Verification items for this drawing (mm, ordinates from the low corner). A direction names the side the tool comes from. Round coordinates to 2 decimals unless told otherwise and drop trailing zeros. Order: outer loops, then holes, each group sorted by start corner. A loop starts at its lowest first (then second) coordinate and runs counter-clockwise, first axis right, second up. Notation, with made-up numbers: (26, -37.5) - (42, -37.5) arc R12 ccw to (42, -32.5) - close; hole circle Ø6 at (48, 21). An arc over 180 degrees is marked (long way). Return JSON: item names as keys, results as strings. Group by question number.
Q1. Sectioned sample at A-A, the plane z = 9.5. Record the cut outline in (x, y).
Q2. Material ranges on line 1 along Y through (x, z) = (3, 14); line 2 along Z through (x, y) = (3.7, 0.5); line 3 along Z through (x, y) = (3.8, 2.35), recorded low to high.
Q3. Tool access check on the marked faces 1 and 2. Record the directions out of +Z, -Z, +X, -X, +Y, -Y that give a thin tool (end or side, any length) a straight path to the whole face; none if there is none.
Q4. Sectioned sample at D-D, the plane y = 4.35. Record the cut outline in (x, z), then the cut area to 3 significant figures.
Q5. Sectioned sample at C-C, the plane y = 2.05. Record the cut outline in (x, z).
Q6. Sectioned sample at B-B, the plane x = 3. Record the cut outline in (y, z).
Q7. Gauge pin test, flat ends, axial feed: pin 1 Ø0.8 at (x, y) = (3, 2.5) entering from -Z; pin 2 Ø2 at (x, y) = (1, 4) entering from +Z. Record the tip position at first contact, or that the pin passes through.
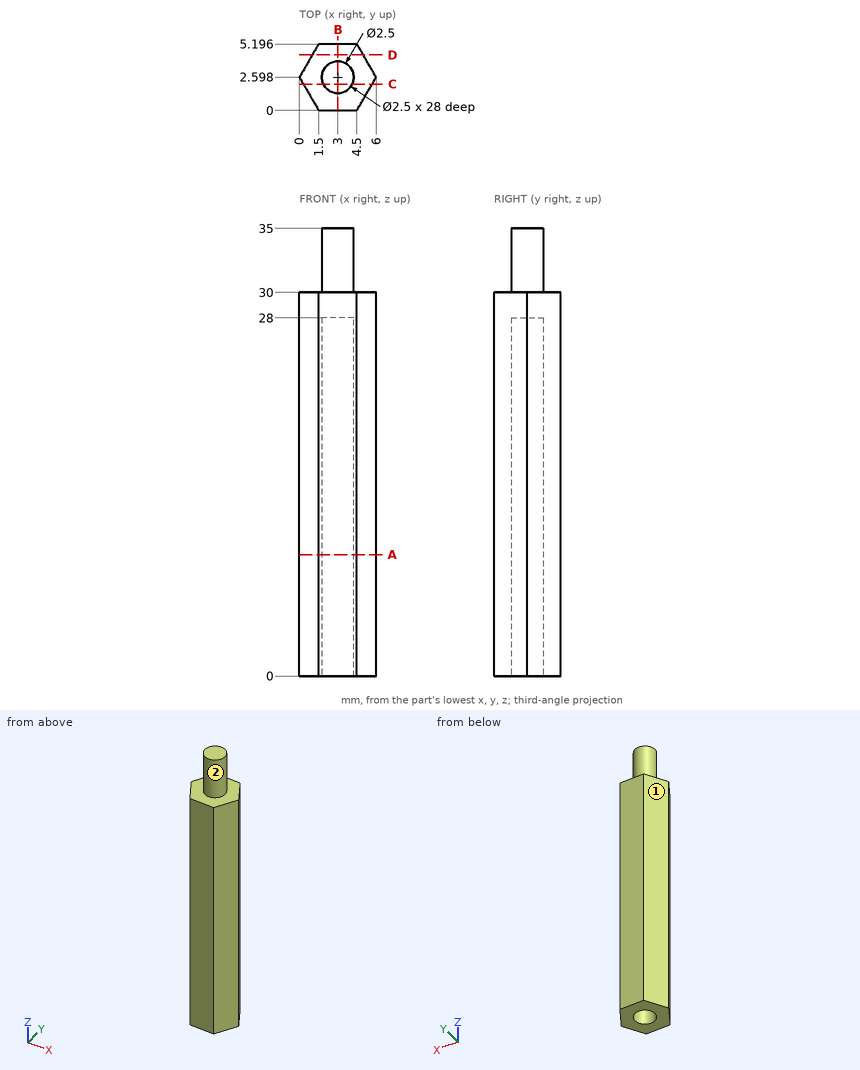
Reply:
{
 "1": {"outline": "(0, 2.6) - (1.5, 0) - (4.5, 0) - (6, 2.6) - (4.5, 5.2) - (1.5, 5.2) - close; hole circle Ø2.5 at (3, 2.6)"},
 "2": {"line 1": "0 to 1.35, 3.85 to 5.2", "line 2": "0 to 30", "line 3": "28 to 35"},
 "3": {"face 1": "+Z, -Z, -X, +Y", "face 2": "+Z"},
 "4": {"outline": "(1.01, 0) - (4.99, 0) - (4.99, 30) - (1.01, 30) - close", "area": "119 mm^2"},
 "5": {"outline": "(0.32, 0) - (1.88, 0) - (1.88, 28) - (4.12, 28) - (4.12, 0) - (5.68, 0) - (5.68, 30) - (4.12, 30) - (4.12, 35) - (1.88, 35) - (1.88, 30) - (0.32, 30) - close"},
 "6": {"outline": "(0, 0) - (1.35, 0) - (1.35, 28) - (3.85, 28) - (3.85, 0) - (5.2, 0) - (5.2, 30) - (3.85, 30) - (3.85, 35) - (1.35, 35) - (1.35, 30) - (0, 30) - close"},
 "7": {"pin 1": "z = 28", "pin 2": "z = 30"}
}
